from build123d import *

# Parameters (mm, degrees)
F0_R     = 17.939821
F0_R_2   = 4.5466
F1_DEPTH = 25.4
F0_R_3   = 41.14561
F2_DEPTH = 12.7
F0_W     = 110.865114
F0_H     = 110.865114
F0_W_2   = 8.71167
F0_H_2   = 20.327227
F3_DEPTH = 12.7
F4_DEPTH = 1.27


with BuildPart() as f1:
    # F0 (on Top) → F1 (new body)
    with BuildSketch(Plane.XY):
        Circle(F0_R)
        Circle(F0_R_2, mode=Mode.SUBTRACT)
    extrude(amount=F1_DEPTH)

    # F0 (on Top) → F2 (join, symmetric)
    with BuildSketch(Plane.XY):
        Circle(F0_R_3)
        Circle(F0_R, mode=Mode.SUBTRACT)
    extrude(amount=F2_DEPTH, both=True)

    # F0 (on Top) → F3 (join)
    with BuildSketch(Plane.XY):
        Rectangle(F0_W, F0_H)
        with Locations((-45.010282, -39.021014)):
            Rectangle(F0_W_2, F0_H_2, mode=Mode.SUBTRACT)
        with Locations((45.010282, -39.021014)):
            Rectangle(F0_W_2, F0_H_2, mode=Mode.SUBTRACT)
        Circle(F0_R_3, mode=Mode.SUBTRACT)
        with Locations((-45.010282, 39.021014)):
            Rectangle(F0_W_2, F0_H_2, mode=Mode.SUBTRACT)
        with Locations((45.010282, 39.021014)):
            Rectangle(F0_W_2, F0_H_2, mode=Mode.SUBTRACT)
    extrude(amount=-F3_DEPTH)

    # F0 (on Top) → F4 (join)
    with BuildSketch(Plane.XY):
        with Locations((-45.010282, 39.021014)):
            Rectangle(F0_W_2, F0_H_2)
        with Locations((45.010282, 39.021014)):
            Rectangle(F0_W_2, F0_H_2)
        with Locations((45.010282, -39.021014)):
            Rectangle(F0_W_2, F0_H_2)
        with Locations((-45.010282, -39.021014)):
            Rectangle(F0_W_2, F0_H_2)
    extrude(amount=-F4_DEPTH)


solid = f1.part
For this review, take the finished solid that the model builds, in its own axes (mm). A direction names the side the tool comes from. Coordinates: 2 decimals unless noted, no trailing zeros. Loops run counter-clockwise (first coordinate to the right, second up) from the corner with the lowest first, then second, coordinate; pieces in that order, holes last. Notation, with made-up numbers: (21, -13) - (45, -13) arc R10 ccw to (45, 1) - close; hole circle Ø6 at (37, -6.75). An arc over 180 degrees is marked (long way). Use a Markdown table: item, result. Add a question column.
Item 1: Mouldability with a two-part tool opening along X and no side actions: class faces 4 (the face through (4, -4, 25.4)), 5 (the face through (-3.351, 3.073, 12.522)), 6 (the face through (9.64, 15.13, 18.96)) as pulls with the +X half, pulls with the -X half, needs draft (parallel to the pull), parting line crosses it, or undercut.
Item 2: We need section A-A (y = 0). Give the boundary of the cut face in (x, z), and give its area (3 significant figures).
Item 3: Tool access review of faces 1 (the face through (-45, 49.185, -7)), 2 (the face through (18, -9, 12.7)), 3 (the face through (-13, 13, -12.7)): name each direction out of +Z, -Z, +X, -X, +Y, -Y from which nothing blocks a thin tool from reaching the whole face with its end or side.
Item 4: Insertion check: pin 1 Ø3 at (y, z) = (1.5, 19.5) entering from +X; pin 2 Ø12 at (x, y) = (0, 0) entering from -Z; pin 3 Ø8 at (x, z) = (-39, 15) entering from -Y; pin 4 Ø5 at (x, z) = (41, 15.5) entering from +Y. Each pin has a flat end and moves straight along its axis. Give the tip position at first contact, or say it passes through.
Item 5: We need section D-D (z = 14.5). Give the boundary of the cut face in (x, y).
Item 6: For line 1 (Y direction, x = -46, z = -6); line 2 (Y direction, x = 0, z = -7); line 3 (Y direction, x = 0, z = 1), list the stretches that pass through material, from the lowest coordinate up.
Item 7: We need section C-C (x = -45). Give the boundary of the cut face in (y, z).
Results list:
| question | item | result |
|---|---|---|
| 1 | face 4 | needs draft |
| 1 | face 5 | undercut |
| 1 | face 6 | parting line crosses it |
| 2 | outline | (-55.43, -12.7) - (-17.94, -12.7) - (-17.94, 0) - (-4.55, 0) - (-4.55, 25.4) - (-17.94, 25.4) - (-17.94, 12.7) - (-41.15, 12.7) - (-41.15, 0) - (-55.43, 0) - close; (4.55, 0) - (17.94, 0) - (17.94, -12.7) - (55.43, -12.7) - (55.43, 0) - (41.15, 0) - (41.15, 12.7) - (17.94, 12.7) - (17.94, 25.4) - (4.55, 25.4) - close |
| 2 | area | 2,220 mm^2 |
| 3 | face 1 | -Z |
| 3 | face 2 | +Z |
| 3 | face 3 | -Z, +X, -X, +Y, -Y |
| 4 | pin 1 | stops at x = 17.94 |
| 4 | pin 2 | stops at z = 0 |
| 4 | pin 3 | stops at y = -20.41 |
| 4 | pin 4 | passes through |
| 5 | outline | circle Ø35.88 at (0, 0); hole circle Ø9.09 at (0, 0) |
| 6 | line 1 | y = -55.43 to -49.18, -28.86 to 28.86, 49.18 to 55.43 |
| 6 | line 2 | y = -55.43 to -17.94, 17.94 to 55.43 |
| 6 | line 3 | y = -41.15 to -4.55, 4.55 to 41.15 |
| 7 | outline | (-55.43, -12.7) - (-49.18, -12.7) - (-49.18, -1.27) - (-28.86, -1.27) - (-28.86, -12.7) - (28.86, -12.7) - (28.86, -1.27) - (49.18, -1.27) - (49.18, -12.7) - (55.43, -12.7) - (55.43, 0) - (-55.43, 0) - close |
